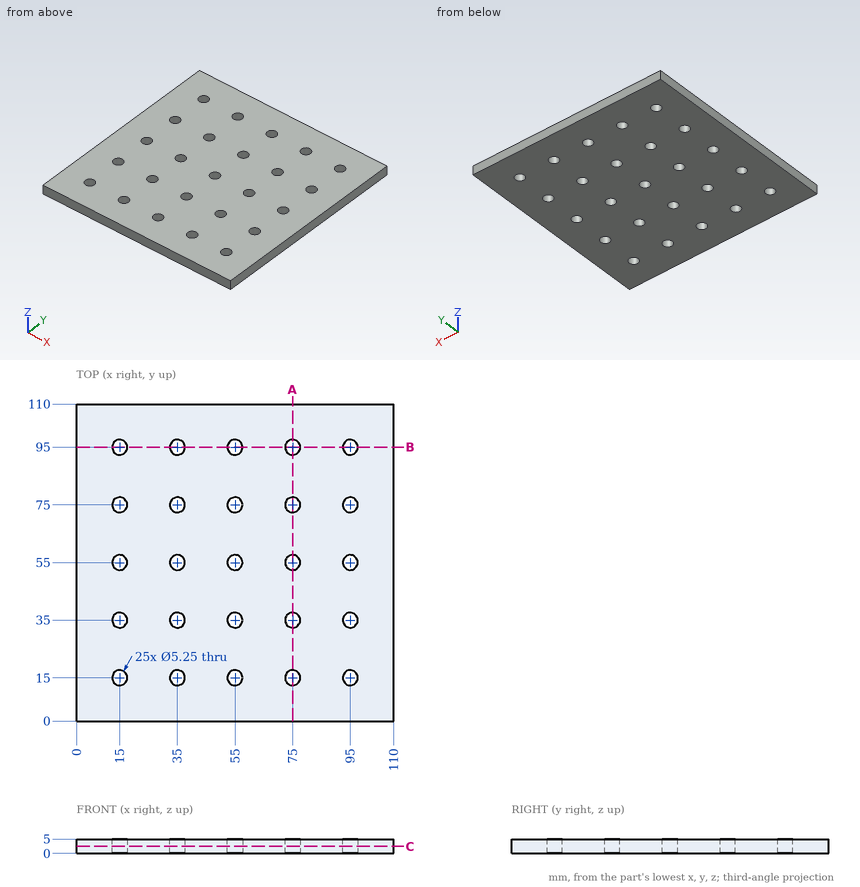
Job drawing, mm, ordinate dimensions from the low corner. One solid piece. Round coordinates to 2 decimals unless told otherwise and drop trailing zeros. Loops run counter-clockwise (first coordinate to the right, second up) from the corner with the lowest first, then second, coordinate; pieces in that order, holes last.
Item 1: Drop a flat-ended pin along its axis: P1, Ø6, axis at x = 35, y = 55, coming from the +Z side. Give the stop position or say it passes through.
Item 2: Drill centre lines: line 1 (X direction, y = 75, z = 2.15) (3 decimals); line 2 (X direction, y = 77, z = 1.85). Where is each one in solid material? Low to high.
Item 3: Cut at C-C, the plane z = 2.45. State how many separate pieces and enclosed holes the cut face has, then the cut area to 3 significant figures.
Item 4: Cut at A-A, the plane x = 75. Give the cut face in (y, z) (3 decimals), then the cut area to 3 significant figures.
A:
1. P1: stops at z = 5
2. line 1: x = 0 to 12.375, 17.625 to 32.375, 37.625 to 52.375, 57.625 to 72.375, 77.625 to 92.375, 97.625 to 110
2. line 2: x = 0 to 13.3, 16.7 to 33.3, 36.7 to 53.3, 56.7 to 73.3, 76.7 to 93.3, 96.7 to 110
3. separate pieces: 1
3. enclosed holes: 25
3. area: 11,600 mm2
4. outline: (0, 0) - (12.375, 0) - (12.375, 5) - (0, 5) - close; (17.625, 0) - (32.375, 0) - (32.375, 5) - (17.625, 5) - close; (37.625, 0) - (52.375, 0) - (52.375, 5) - (37.625, 5) - close; (57.625, 0) - (72.375, 0) - (72.375, 5) - (57.625, 5) - close; (77.625, 0) - (92.375, 0) - (92.375, 5) - (77.625, 5) - close; (97.625, 0) - (110, 0) - (110, 5) - (97.625, 5) - close
4. area: 419 mm2
